```python
from build123d import *

# Parameters (mm, degrees)
F0_W     = 96
F0_H     = 64
F0_R     = 10
F1_DEPTH = 20
F5_DEPTH = 6
F6_DEPTH = 18
F8_R     = 15


with BuildPart() as f1:
    # F0 (on Top) → F1 (new body)
    with BuildSketch(Plane.XY):
        Rectangle(F0_W, F0_H)
        with Locations((-28, 0)):
            Circle(F0_R, mode=Mode.SUBTRACT)
        with Locations((28, 0)):
            Circle(F0_R, mode=Mode.SUBTRACT)
    extrude(amount=-F1_DEPTH)


with BuildPart() as f3:
    # F2 (on Right) → F3 (revolve)
    with BuildSketch(Plane.YZ):
        Polygon((50.3847763109, 144.3847763109), (43.313708499, 137.313708499), (65.941125497, 114.686291501), (73.0121933088, 121.7573593129), align=None)
        Polygon((73.0121933088, 121.7573593129), (65.941125497, 114.686291501), (74.4264068712, 106.2010101268), (85.7401153702, 117.5147186258), (77.2548339959, 126), align=None)
    revolve(axis=Axis((0, 47.5563491861, 110.4436508139), (0, 0.7071067812, -0.7071067812)))


with BuildPart() as f5:
    # F4 (on Right) → F5 (new body, symmetric)
    with BuildSketch(Plane.YZ):
        Polygon((9.5233405971, 95.0380592229), (27.908116908, 76.653282912), (40.7393130211, 89.4844790252), (22.3545367103, 107.869255336), align=None)
        with BuildLine():
            Line((-32, 0), (20, 0))
            Line((20, 0), (20, 57.56139982))
            ThreePointArc((20, 57.56139982), (22.0552526222, 67.8938524938), (27.908116908, 76.653282912))
            Line((27.908116908, 76.653282912), (9.5233405971, 95.0380592229))
            ThreePointArc((9.5233405971, 95.0380592229), (-1.9656152231, 77.8436217353), (-6, 57.56139982))
            ThreePointArc((-6, 57.56139982), (-12.9154073667, 30.2063601077), (-32, 9.4241710813))
            Line((-32, 9.4241710813), (-32, 0))
        make_face()
    extrude(amount=F5_DEPTH, both=True)


with BuildPart() as f6:
    # F4 (on Right) → F6 (new body, symmetric)
    with BuildSketch(Plane.YZ):
        with BuildLine():
            Line((20, 0), (32, 0))
            Line((32, 0), (32, 57.56139982))
            ThreePointArc((32, 57.56139982), (33.1418070123, 63.3016513055), (36.3933982822, 68.1680015378))
            Line((36.3933982822, 68.1680015378), (27.908116908, 76.653282912))
            ThreePointArc((27.908116908, 76.653282912), (22.0552526222, 67.8938524938), (20, 57.56139982))
            Line((20, 57.56139982), (20, 0))
        make_face()
        Polygon((27.908116908, 76.653282912), (36.3933982822, 68.1680015378), (49.2245943954, 80.9991976509), (40.7393130211, 89.4844790252), align=None)
    extrude(amount=F6_DEPTH, both=True)

    # F7: union F1, F3, F5
    add(f1.part)
    add(f3.part)
    add(f5.part)

    # F8
    f8_edges = [f6.edges().sort_by_distance(p)[0] for p in [
        (18, 40.161771, 80.421655),
        (-18, 40.161771, 80.421655),
    ]]
    fillet(f8_edges, radius=F8_R)


solid = f6.part
```
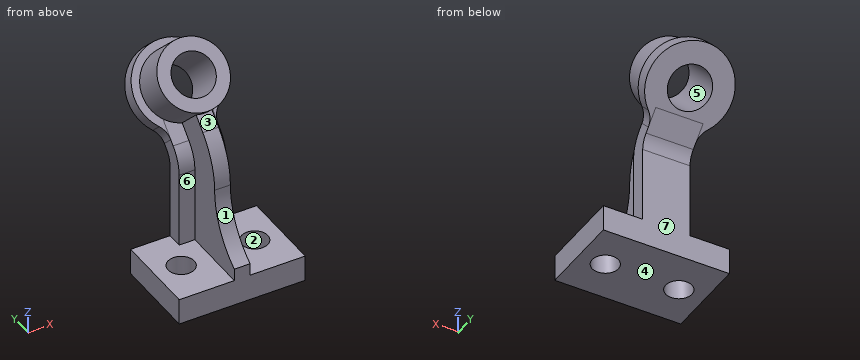
Can you work these out from the model? Positions are in its coordinate system, mm. Face numbers are marked on the shaded views. A direction names the side the tool comes from. Coordinates: 2 decimals unless noted, no trailing zeros. Order: outer loops, then holes, each group sorted by start corner. A loop starts at its lowest first (then second) coordinate and runs counter-clockwise, first axis right, second up.
1. I'm going to push flat-ended pins straight in: pin 1 (8 mm diameter, centred on y = 13.5, z = 59.5, fed in from +X); pin 2 (18 mm diameter, centred on x = -28, y = 0, fed in from -Z); pin 3 (21.5 mm diameter, centred on y = 28, z = 31, fed in from +X); pin 4 (3 mm diameter, centred on x = -15.5, z = 12.5, fed in from -Y). Where does each tip first touch, or does it pass through?
2. If we section it at C-C (y = 0): Please give me the cut outline in (x, z).
3. If we section it at A-A (x = 28): Please give me the cut outline in (y, z), then the cut area to 3 significant figures.
4. If we section it at D-D (x = -11.5): Please give me the cut outline in (y, z), then the cut area to 3 significant figures.
5. If we section it at B-B (z = -6): Please give me the cut outline in (x, y).
6. I need wall thicknesses on line 1 (X direction, y = -4, z = -0.5); line 2 (Y direction, x = 28, z = -6.25); line 3 (Z direction, x = 26, y = -21). Which ranges of each line are inside material? Lowest first, please.
7. Thinking about a two-plate mould opening in Z: for the marked faces 1, 2, 3 and 4, which applies, +Z half, -Z half, draft (parallel to the pull), parting line (faces both ways), or undercut?
8. For the marked faces 5, 6 and 7, which set-ups out of +Z, -Z, +X, -X, +Y, -Y let a thin tool reach every point of the face, with its end or its side?
Entries:
1. pin 1: stops at x = 6
1. pin 2: passes through
1. pin 3: stops at x = 18
1. pin 4: stops at y = 20
2. outline: (-48, -20) - (-38, -20) - (-38, 0) - (-48, 0) - close; (-18, -20) - (18, -20) - (18, 0) - (6, 0) - (6, 82.06) - (-6, 82.06) - (-6, 0) - (-18, 0) - close; (38, -20) - (48, -20) - (48, 0) - (38, 0) - close
3. outline: (-32, -20) - (-10, -20) - (-10, 0) - (-32, 0) - close; (10, -20) - (32, -20) - (32, 0) - (10, 0) - close; (43.67, 92.42) - (52.16, 83.93) - (74.07, 105.84) - (65.58, 114.33) - close
3. area: 1,250 mm2
4. outline: (-32, -20) - (32, -20) - (32, 57.56) arc R15 cw to (36.39, 68.17) - (55.25, 87.02) - (24.13, 118.13) - (15.51, 109.51) - (38.14, 86.88) - (27.91, 76.65) arc R27 ccw to (20, 57.56) - (20, 0) - (-32, 0) - close; (39.87, 133.87) - (70.98, 102.75) - (84.23, 116) - (75.74, 124.49) - (71.12, 119.86) - (48.49, 142.49) - close
4. area: 3,490 mm2
5. outline: (-48, -32) - (48, -32) - (48, 32) - (-48, 32) - close; hole circle Ø20 at (-28, 0); hole circle Ø20 at (28, 0)
6. line 1: x = -48 to -37.17, -18.83 to 18.83, 37.17 to 48
6. line 2: y = -32 to -10, 10 to 32
6. line 3: z = -20 to 0
7. face 1: +Z half
7. face 2: draft
7. face 3: undercut
7. face 4: -Z half
8. face 5: none
8. face 6: -X, -Y
8. face 7: -Z, +X, -X, +Y
